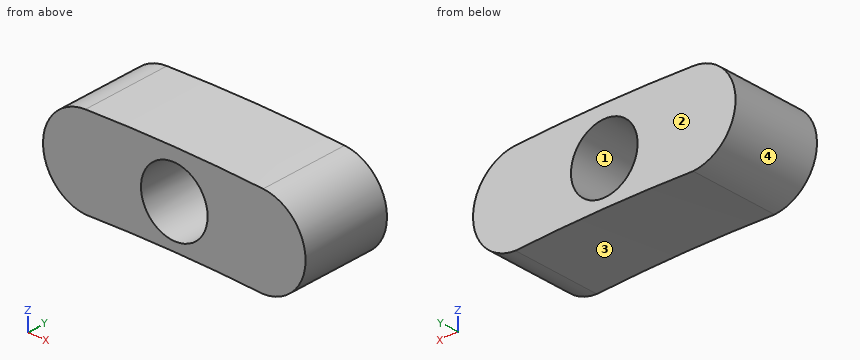
from build123d import *

# Parameters (mm, degrees)
F0_R     = 2.38125
F1_DEPTH = 6.35


with BuildPart() as f1:
    # F0 (on Front) → F1 (new body)
    with BuildSketch(Plane.XZ):
        with BuildLine():
            ThreePointArc((-6.35, 0), (0, 0.146256), (6.35, 0))
            ThreePointArc((6.35, 0), (9.382037, 3.175), (6.35, 6.35))
            ThreePointArc((6.35, 6.35), (0, 6.496256), (-6.35, 6.35))
            ThreePointArc((-6.35, 6.35), (-9.382037, 3.175), (-6.35, 0))
        make_face()
        with Locations((0, 3.175)):
            Circle(F0_R, mode=Mode.SUBTRACT)
    extrude(amount=F1_DEPTH)


solid = f1.part
Input: part model. Units: mm. Frame: model coordinates. Face numbers are marked on the shaded views. Give positions to 0.01 mm unless a question says otherwise; leave off trailing zeros. Write each loop counter-clockwise with the first axis right and the second up, starting at its lowest first coordinate (ties: lowest second). Pieces come first, ordered by that corner, then holes. Notation, with made-up numbers: M 44,52.5 L 76,52.5 A28 cw 76,81.5 Z; hole C 2.5,80.5 d3. An arc over 180 degrees is marked long. Write item = value, one per line. Start each with the question number.
1) Cut plane B-B on z = 1.25. Return the cut outline in (x, y).
2) Cut plane D-D on x = -7.5. Return the cut outline in (y, z).
3) Material intervals for line 1 along X through (y, z) = (-1.5, 2.5); line 2 along X through (y, z) = (-1.5, 3.5); line 3 along Z through (x, y) = (1.75, -3.75), sorted ascending. Write a range as [from, to].
4) First-contact query: pin 1 Ø1.5 at (y, z) = (-3, 4.5) entering from -X; pin 2 Ø2 at (y, z) = (-4, 4.5) entering from -X. Flat tips, straight axial feed; report the tip coordinate or a pass-through.
5) Draft query along X for the marked faces 1, 2, 3 and 4. Return one class per face: +X half, -X half, draft (parallel to the pull), parting line (faces both ways), or undercut.
6) Cut plane A-A on x = 0. Return the cut outline in (y, z), then the cut area to 3 significant figures.
Solved:
q1.outline = M -8.73,-6.35 L -1.4,-6.35 L -1.4,0 L -8.73,0 Z; M 1.4,-6.35 L 8.73,-6.35 L 8.73,0 L 1.4,0 Z
q2.outline = M -6.35,0.27 L 0,0.27 L 0,6.08 L -6.35,6.08 Z
q3.line_1 = [-9.31, -2.28], [2.28, 9.31]
q3.line_2 = [-9.37, -2.36], [2.36, 9.37]
q3.line_3 = [0.14, 1.56], [4.79, 6.49]
q4.pin_1 = -9.33
q4.pin_2 = -9.37
q5.face_1 = undercut
q5.face_2 = draft
q5.face_3 = undercut
q5.face_4 = -X half
q6.outline = M -6.35,0.15 L 0,0.15 L 0,0.79 L -6.35,0.79 Z; M -6.35,5.56 L 0,5.56 L 0,6.5 L -6.35,6.5 Z
q6.area = 10.1 mm2
